Can you work these out from the model? Positions are in its coordinate system, mm. Face numbers are marked on the shaded views. A direction names the side the tool comes from. Give positions to 0.01 mm unless a question says otherwise; leave off trailing zeros. Write each loop counter-clockwise with the first axis right and the second up, starting at its lowest first coordinate (ties: lowest second). Pieces come first, ordered by that corner, then holes. Notation, with made-up numbers: (-6.5, -33) -> (50.5, -33) arc R22 ccw to (50.5, -22) -> close; hole circle Ø11 at (60.5, 8). An arc over 180 degrees is marked (long way). Answer as CSV lines item,"result". Start each with the question number.
1. If we section it at A-A on z = 24: Write out the boundary of the cut face in (x, y), plus the area to 3 significant figures.
2. If we section it at C-C on y = 3: Write out the boundary of the cut face in (x, z), plus the area to 3 significant figures.
3. I need wall thicknesses on line 1 (Y direction, x = -2.5, z = 7); line 2 (Z direction, x = 40.5, y = -4.5); line 3 (X direction, y = -8.5, z = 47). Which ranges of each line are inside material? Lowest first, please. Write a range as [from, to].
4. If we section it at B-B on x = -28: Write out the boundary of the cut face in (y, z), plus the area to 3 significant figures.
5. If we section it at D-D on x = -2.5: Write out the boundary of the cut face in (y, z), plus the area to 3 significant figures.
6. On a 3-axis mill with a long thin cutter (end or side, diameter ignored), from which of +Z, -Z, +X, -X, +Y, -Y can I reach the whole of each face in a straight line? I mean the marked faces 1, 2 and 3. Say none if no direction works.
7. I'm going to push flat-ended pins straight in: P1, Ø3, axis at x = -15.5, y = -3, coming from the +Z side; P2, Ø11.5, axis at x = -2.5, y = -25, coming from the +Z side; P3, Ø24, axis at y = -36, z = 23.5, coming from the +X side. Where does each tip first touch, or does it pass through?
8. If we mould it in two halves opening along Y, with no side actions, what happens to the marked faces 4, 5 and 6? For each: pulls with the +Y half, pulls with the -Y half, needs draft (parallel to the pull), parting line crosses it, or undercut.
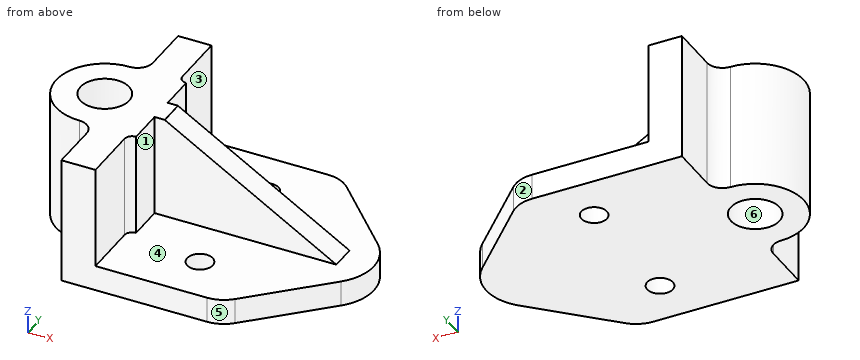
Autodesk Fusion 360 part; units mm, degrees
sketch "Sketch1" plane through (0, 0, 0) normal (0, 0, 1) x (1, 0, 0)
  line L0 (9.969, -44) -> (-33.5, -44)
  line L1 (-33.5, -44) -> (-33.5, 44)
  line L2 (-33.5, 44) -> (11.9673, 44)
  arc A0 (46.682, -13.6834) -> (47.1834, 13.182) centre (33.5, 0) ccw
  line L3 (46.682, -13.6834) -> (18.9882, -40.3623)
  line L4 (47.1834, 13.182) -> (21.3296, 40.0192)
  circle A1 centre (-2.5, 25) radius 5
  circle A2 centre (-2.5, -25) radius 5
  arc A3 (21.3296, 40.0192) -> (11.9673, 44) centre (11.9673, 31) ccw
  line L5 (33.5, 27.3859) -> (33.5, 25)
  line L6 (33.5, -25) -> (33.5, -26.3823)
  line L7 (-2.5, -25) -> (-1.5636, -25) construction
  arc A4 (9.969, -44) -> (18.9882, -40.3623) centre (9.969, -31) ccw
  dimension "d4" = 88
  dimension "d6" = 19
  dimension "d10" = 10
  dimension "d11" = 10
extrude "Extrude1" add sketch "Sketch1" along normal blind 10 makes body 1
sketch "Sketch2" plane through (0, 0, 10) normal (0, 0, 1) x (-1, 0, 0)
  circle A0 centre (2.5, -25) radius 5
  circle A1 centre (2.5, 25) radius 5
  line L0 (33.5, 44) -> (-9.969, 44)
  arc A2 (-9.969, 44) -> (-18.9882, 40.3623) centre (-9.969, 31) ccw
  line L1 (-18.9882, 40.3623) -> (-46.682, 13.6834)
  arc A3 (-46.682, 13.6834) -> (-47.1834, -13.182) centre (-33.5, 0) ccw
  line L2 (-47.1834, -13.182) -> (-21.3296, -40.0192)
  arc A4 (-21.3296, -40.0192) -> (-11.9673, -44) centre (-11.9673, -31) ccw
  line L3 (-11.9673, -44) -> (33.5, -44)
  line L4 (33.5, -44) -> (33.5, 44)
  line L5 (46.8066, 44) -> (33.5, 44)
  line L6 (30.5, 19) -> (30.5, 5)
  line L7 (30.5, 5) -> (26.5, 5)
  line L8 (26.5, 5) -> (26.5, -5)
  line L9 (26.5, -5) -> (30.5, -5)
  line L10 (30.5, -5) -> (30.5, -19)
  line L11 (33.5, -44) -> (46.5, -44)
  line L12 (33.5, 0) -> (52.4999, -0.0662) construction
  circle A5 centre (52.4999, -0.0662) radius 9.5
  line L13 (46.5, -44) -> (46.566, -25.0452)
  line L14 (46.7402, 24.9536) -> (46.8066, 44)
  arc A6 (52.5501, -19.0661) -> (52.6825, 18.9329) centre (52.4999, -0.0662) ccw
  arc A7 (33.5, 0) -> (33.5, -0.1324) centre (52.4999, -0.0662) ccw
  arc A8 (52.5501, -19.0661) -> (46.566, -25.0452) centre (52.566, -25.0661) ccw
  arc A9 (46.7402, 24.9536) -> (52.6825, 18.9329) centre (52.7402, 24.9327) ccw
  arc A10 (33.5, -22) -> (30.5, -19) centre (30.5, -22) ccw
  arc A11 (30.5, 19) -> (33.5, 22) centre (30.5, 22) ccw
  dimension "d17" = 4
  dimension "d19" = 38
  dimension "d21" = 13
  dimension "d22" = 10
  dimension "d23" = 14
  dimension "d25" = 19
  dimension "d27" = 19
  dimension "d28" = 6
  dimension "d29" = 6
  dimension "d30" = 3
  dimension "d31" = 3
extrude "Extrude2" add sketch "Sketch2" against normal blind 10 separate body contours L4 L5 L11 L13 L14 A6 A7 A8 A9 | L4 L6 L7 L8 L9 L10 A7 A10 A11 makes body 2
extrude "Extrude3" add 1 faces at (-37.9134, -30.3179, 10) along direction (0, 0, 1) blind 30 on bodies 2 bodies 2 1
extrude "Extrude5" add 1 faces at (-37.9134, -30.3179, 40) along direction (0, 0, 1) blind 10 on bodies 2 bodies 2
sketch "Sketch4" plane through (0, 0, 0) normal (0, 1, 0) x (1, 0, 0)
  line L0 (-26.5123, -49.9551) -> (-26.5123, -9.9551)
  line L1 (-26.5123, -9.9551) -> (40.4877, -9.9551)
  line L2 (40.4877, -9.9551) -> (-26.5123, -49.9551)
  line L3 (-26.5, -10) -> (-26.5, -50)
  dimension "d43" = 40
  dimension "d44" = 67
  dimension "d45" = 40
extrude "Extrude6" add sketch "Sketch4" along normal mid plane 10 bodies 2
Computed values:
1,outline,"(-52.68, -18.93) arc R6 cw to (-46.74, -24.95) -> (-46.81, -44) -> (-33.5, -44) -> (-33.5, -22) arc R3 cw to (-30.5, -19) -> (-30.5, -5) -> (16.96, -5) -> (16.96, 5) -> (-30.5, 5) -> (-30.5, 19) arc R3 cw to (-33.5, 22) -> (-33.5, 44) -> (-46.5, 44) -> (-46.57, 25.05) arc R6 cw to (-52.55, 19.07) arc R19 ccw to start; hole circle Ø19 at (-52.5, 0.07)"
1,area,"2,270 mm2"
2,outline,"(-71.27, 0) -> (-61.54, 0) -> (-61.54, 50) -> (-71.27, 50) -> close; (-43.46, 0) -> (52.26, 0) -> (52.26, 10) -> (40.41, 10) -> (-26.5, 49.95) -> (-26.5, 50) -> (-43.46, 50) -> close"
2,area,"3,460 mm2"
3,line 1,"y = [-44, -30], [-20, 20], [30, 44]"
3,line 2,"z = [0, 10]"
3,line 3,"x = [-69.46, -56.61], [-48.39, -30.5]"
4,outline,"(-44, 0) -> (44, 0) -> (44, 10) -> (5, 10) -> (5, 50) -> (-5, 50) -> (-5, 10) -> (-44, 10) -> close"
4,area,"1,280 mm2"
5,outline,"(-44, 0) -> (-30, 0) -> (-30, 10) -> (-44, 10) -> close; (-20, 0) -> (20, 0) -> (20, 10) -> (5, 10) -> (5, 35.62) -> (-5, 35.62) -> (-5, 10) -> (-20, 10) -> close; (30, 0) -> (44, 0) -> (44, 10) -> (30, 10) -> close"
5,area,"936 mm2"
6,face 1,"+Z, +X, -Y"
6,face 2,"+Z, -Z, +X, +Y"
6,face 3,"+Z, +X, +Y"
7,P1,"stops at z = 44.28"
7,P2,"stops at z = 10"
7,P3,"stops at x = -33.5"
8,face 4,"needs draft"
8,face 5,"pulls with the -Y half"
8,face 6,"undercut"
